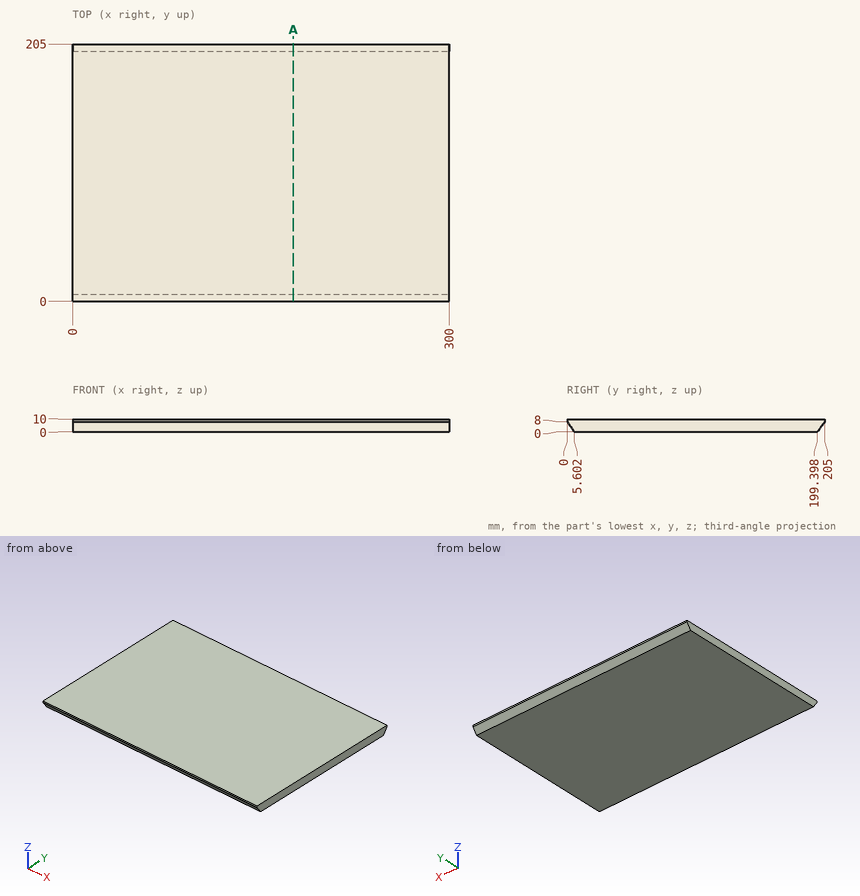
Design review of the part shown in the three views and the two pictorial views. Dimensions are in mm from the part's minimum x, y and z. Give positions to 0.01 mm unless a question says otherwise; leave off trailing zeros. Loops run counter-clockwise (first coordinate to the right, second up) from the corner with the lowest first, then second, coordinate; pieces in that order, holes last. Notation, with made-up numbers: (72, 42) -> (113, 42) arc R19 cw to (113, 57) -> close; hole circle Ø1 at (86.25, 85.5). An arc over 180 degrees is marked (long way). Answer as a JSON object with one key per item and string values. Group by question number.
Q1. Wall thickness on line 1 along Y through (x, z) = (278, 1.5); line 2 along Y through (x, z) = (272.5, 5.5): over which ranges is each line inside the solid? List them lowest first.
Q2. Take a section at A-A (x = 176). Write out the cut boundary in (y, z), plus the area to 4 significant figures.
Q3. Insertion check: pin 1 (2 mm diameter, centred on x = 262, z = 5.5, fed in from +Y); pin 2 (2 mm diameter, centred on x = 166.5, z = 3.5, fed in from -Y). Each pin has a flat end and moves straight along its axis. Give the tip position at first contact, or say it passes through.
Answer below:
{
 "1": {"line 1": "y = 4.55 to 200.45", "line 2": "y = 1.75 to 203.25"},
 "2": {"outline": "(0, 8) -> (5.6, 0) -> (199.4, 0) -> (205, 8) -> (205, 10) -> (0, 10) -> close", "area": "2,005 mm2"},
 "3": {"pin 1": "stops at y = 203.95", "pin 2": "stops at y = 2.45"}
}
